The model under review builds one solid part; all positions refer to its coordinate system, in mm. A direction names the side the tool comes from. Give positions to 0.01 mm unless a question says otherwise; leave off trailing zeros. Loops run counter-clockwise (first coordinate to the right, second up) from the corner with the lowest first, then second, coordinate; pieces in that order, holes last. Notation, with made-up numbers: M 70.5,74.25 L 116.5,74.25 A24 cw 116.5,112.25 Z; hole C 37.25,49.25 d7. An arc over 180 degrees is marked long. Return JSON: item names as keys, results as strings. Group by question number.
```python
from build123d import *

# Parameters (mm, degrees)
F0_R          = 50.8
F0_R_2        = 7.9375
F1_DEPTH      = 4.5
F1_DEPTH_BACK = 5
F2_R          = 40.8
F2_R_2        = 7.9375
F3_DEPTH      = 4
F4_W          = 6.35
F4_H          = 6.35
F5_DEPTH      = 17.001


# Not quite as in the source:
# - a pattern or mirror of a feature is missing from the dataset's text; its kind, count and spacing are read off the source's solid


with BuildPart() as f1:
    # F0 (on Top) → F1 (new body, two sides)
    with BuildSketch(Plane.XY) as f1_sk:
        Circle(F0_R)
        Circle(F0_R_2, mode=Mode.SUBTRACT)
    extrude(amount=F1_DEPTH)
    extrude(f1_sk.sketch, amount=-F1_DEPTH_BACK)

    # F2 (on face) → F3 (join)
    with BuildSketch(Plane.XY.offset(4.5)):
        Circle(F2_R)
        Circle(F2_R_2, mode=Mode.SUBTRACT)
    f3 = extrude(amount=F3_DEPTH)

    # F3_copies: F3 across plane
    add(f3.mirror(Plane(origin=(0, 0, 0), x_dir=(-1, 0, 0), z_dir=(0, 0, -1))))

    # F4 (on face) → F5 (cut, through all)
    with BuildSketch(Plane.XY.offset(8.5)):
        with Locations((0, 7.9375)):
            Rectangle(F4_W, F4_H)
    extrude(amount=-F5_DEPTH, mode=Mode.SUBTRACT)


solid = f1.part
```
(1) For faces 1 (the flat face through (-0.6, -8.5, -8.5)), 2 (the flat face through (0, 42, 4.5)), 3 (the flat face through (0, 11.112, 0)), 4 (the flat face through (0, 42, -5)), list the 3-axis set-ups (+Z, -Z, +X, -X, +Y, -Y) from which the entire face can be reached by the end or side of a thin tool; tool diameter is ignored.
(2) For probe 1 along Y at (x, z) = (0, 0.5); probe 2 along Z at (x, y) = (-43, -11); probe 3 along X at (y, z) = (-2.5, 5.5), list the stretches that pass through material, from the lowest coordinate up.
(3) Add section A-A (x = 0). Write out the cut boundary in (y, z).
(4) For pin 1 (1.9 mm diameter, centred on y = 9, z = 1.5, fed in from +X); pin 2 (5 mm diameter, centred on x = -1, z = -3.5, fed in from -Y); pin 3 (14.5 mm diameter, centred on x = 0, y = 0, fed in from +Z); pin 4 (1.2 mm diameter, centred on y = 8.5, z = 2, fed in from -X), all flat-tipped, find the tip position at first contact; note any pin that passes through.
(5) Add section D-D (x = -11). Write out the cut boundary in (y, z).
(6) Add section C-C (z = 7). Write out the cut boundary in (x, y) (1 decimal), and give its area (3 significant figures).
(7) Mouldability with a two-part tool opening along Y and no side actions: class faces 5 (the cylindrical face through (18.827, -36.197, 6.472)), 6 (the cylindrical face through (-0.3, -7.93, -0.12)), 7 (the flat face through (-0.6, -8.5, 8.5)) as released by +Y, released by -Y, zero draft, split by the parting line, or undercut.
(8) Add section B-B (y = 0). Write out the cut boundary in (x, z), and give its area (3 significant figures).
Verdict:
{
 "1": {"face 1": "-Z, +X, -X, +Y, -Y", "face 2": "+Z", "face 3": "+Z, -Z", "face 4": "-Z"},
 "2": {"probe 1": "y = -50.8 to -7.94, 11.11 to 50.8", "probe 2": "z = -5 to 4.5", "probe 3": "x = -40.72 to -7.53, 7.53 to 40.72"},
 "3": {"outline": "M -50.8,-5 L -40.8,-5 L -40.8,-8.5 L -7.94,-8.5 L -7.94,8.5 L -40.8,8.5 L -40.8,4.5 L -50.8,4.5 Z; M 11.11,-8.5 L 40.8,-8.5 L 40.8,-5 L 50.8,-5 L 50.8,4.5 L 40.8,4.5 L 40.8,8.5 L 11.11,8.5 Z"},
 "4": {"pin 1": "stops at x = 50.16", "pin 2": "stops at y = -50.8", "pin 3": "passes through", "pin 4": "stops at x = -50.18"},
 "5": {"outline": "M -49.59,-5 L -39.29,-5 L -39.29,-8.5 L 39.29,-8.5 L 39.29,-5 L 49.59,-5 L 49.59,4.5 L 39.29,4.5 L 39.29,8.5 L -39.29,8.5 L -39.29,4.5 L -49.59,4.5 Z"},
 "6": {"outline": "C 0,0 d81.6; hole M -3.2,7.3 A7.9 ccw long 3.2,7.3 L 3.2,11.1 L -3.2,11.1 Z", "area": "5,010 mm²"},
 "7": {"face 5": "split by the parting line", "face 6": "undercut", "face 7": "zero draft"},
 "8": {"outline": "M -50.8,-5 L -40.8,-5 L -40.8,-8.5 L -7.94,-8.5 L -7.94,8.5 L -40.8,8.5 L -40.8,4.5 L -50.8,4.5 Z; M 7.94,-8.5 L 40.8,-8.5 L 40.8,-5 L 50.8,-5 L 50.8,4.5 L 40.8,4.5 L 40.8,8.5 L 7.94,8.5 Z", "area": "1,310 mm²"}
}
